Verification items for this drawing (mm, ordinates from the low corner). Round coordinates to 2 decimals unless told otherwise and drop trailing zeros. Order: outer loops, then holes, each group sorted by start corner. A loop starts at its lowest first (then second) coordinate and runs counter-clockwise, first axis right, second up. Notation, with made-up numbers: (74.5, -35) -> (78.5, -35) arc R12 cw to (78.5, -26) -> close; hole circle Ø11 at (-26, 46.5). An arc over 180 degrees is marked (long way). Put each result on its own line as item: value.
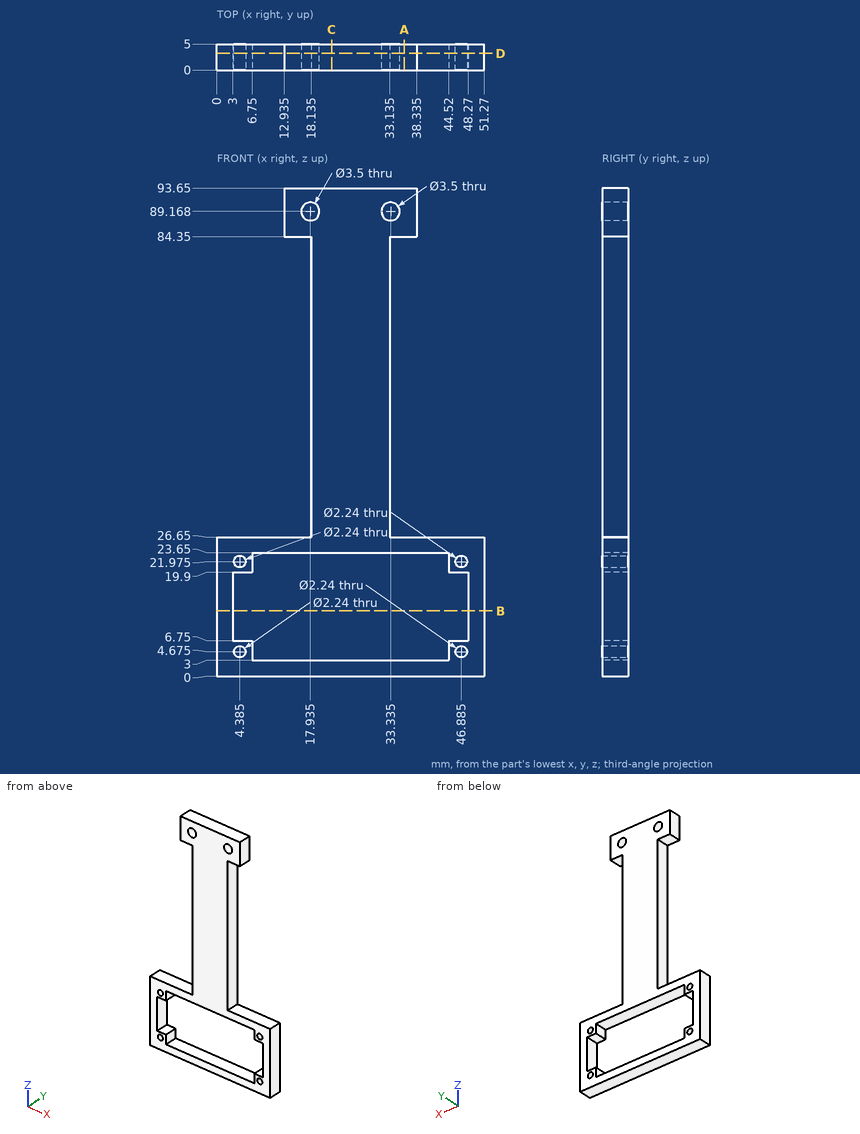
Item 1: Material ranges on L1, parallel to Z at x = 15, y = 2.75; L2, parallel to Z at x = 47, y = 1.95; L3, parallel to Z at x = 12.5, y = 4.35, recorded low to high. Write a range as [from, to].
Check sheet entries:
L1: z = [0, 3], [23.65, 26.65], [84.35, 93.65]
L2: z = [0, 3.56], [5.79, 6.75], [19.9, 20.86], [23.09, 26.65]
L3: z = [0, 3], [23.65, 26.65]
Item 2: Gauge pin test, flat end, axial feed: pin 1 Ø10 at (x, z) = (42.5, 33.5) entering from -Y. Record the tip position at first contact, or that the pin passes through.
Check sheet entries:
pin 1: passes through
Item 3: Section check B-B on z = 12.5. Record the boundary of the cut face in (x, y), then the cut area to 3 significant figures.
Check sheet entries:
outline: (0, 0) -> (3, 0) -> (3, 5) -> (0, 5) -> close; (48.27, 0) -> (51.27, 0) -> (51.27, 5) -> (48.27, 5) -> close
area: 30.0 mm^2
Item 4: Section check A-A on x = 36. Record the boundary of the cut face in (y, z), then the cut area to 3 significant figures.
Check sheet entries:
outline: (0, 0) -> (5, 0) -> (5, 3) -> (0, 3) -> close; (0, 23.65) -> (5, 23.65) -> (5, 26.65) -> (0, 26.65) -> close; (0, 84.35) -> (5, 84.35) -> (5, 93.65) -> (0, 93.65) -> close
area: 76.5 mm^2
Item 5: Section check C-C on x = 22. Record the boundary of the cut face in (y, z).
Check sheet entries:
outline: (0, 0) -> (5, 0) -> (5, 3) -> (0, 3) -> close; (0, 23.65) -> (5, 23.65) -> (5, 93.65) -> (0, 93.65) -> close
Item 6: Section check D-D on y = 3.2. State how many separate pieces and enclosed holes the cut face has, then the cut area to 3 significant figures.
Check sheet entries:
separate pieces: 1
enclosed holes: 7
area: 1,550 mm^2
